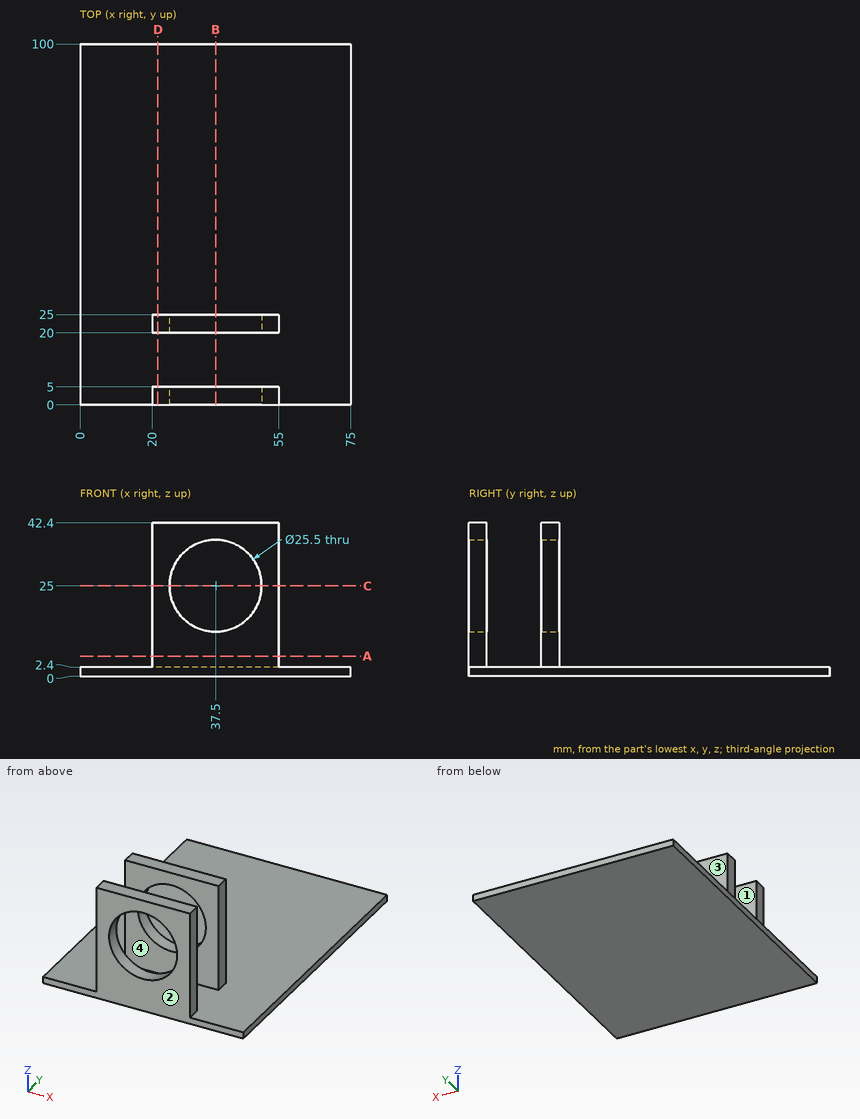
Geometry: see drawing. Coordinates: mm, zero at the bounding-box minimum. Coordinates: 2 decimals unless noted, no trailing zeros. Loops run counter-clockwise (first coordinate to the right, second up) from the corner with the lowest first, then second, coordinate; pieces in that order, holes last. Notation, with made-up numbers: (37, 33) -> (64, 33) arc R20 ccw to (64, 50) -> close; hole circle Ø8 at (-39, -18). An arc over 180 degrees is marked (long way). Use a Markdown table: item, result.
1) Contact query for flat-ended pins moving along their axis: pin 1 (5.5 mm diameter, centred on y = 2.5, z = 31, fed in from +X); pin 2 (22.5 mm diameter, centred on x = 20.5, y = 68, fed in from +Z); pin 3 (6 mm diameter, centred on x = 40, z = 18, fed in from +Y); pin 4 (4 mm diameter, centred on y = 22.5, z = 21.5, fed in from -X). Output: stop coordinate, or through.
Results found:
| item | result |
|---|---|
| pin 1 | stops at x = 55 |
| pin 2 | stops at z = 2.4 |
| pin 3 | passes through |
| pin 4 | stops at x = 20 |
2) Cut plane A-A (z = 5.5). Return the cut outline in (x, y).
Results found:
| item | result |
|---|---|
| outline | (20, 0) -> (55, 0) -> (55, 5) -> (20, 5) -> close; (20, 20) -> (55, 20) -> (55, 25) -> (20, 25) -> close |
3) Cut plane B-B (x = 37.5). Return the cut outline in (y, z), then the cut area to 3 significant figures.
Results found:
| item | result |
|---|---|
| outline | (0, 0) -> (100, 0) -> (100, 2.4) -> (25, 2.4) -> (25, 12.25) -> (20, 12.25) -> (20, 2.4) -> (5, 2.4) -> (5, 12.25) -> (0, 12.25) -> close; (0, 37.75) -> (5, 37.75) -> (5, 42.4) -> (0, 42.4) -> close; (20, 37.75) -> (25, 37.75) -> (25, 42.4) -> (20, 42.4) -> close |
| area | 385 mm2 |
4) Material intervals for line 1 along Z through (x, y) = (37, 1); line 2 along X through (y, z) = (22.8, 25); line 3 along Y through (x, z) = (24.5, 30.5), sorted ascending. Write a range as from..to.
Results found:
| item | result |
|---|---|
| line 1 | z = 0..12.26, 37.74..42.4 |
| line 2 | x = 20..24.75, 50.25..55 |
| line 3 | y = 0..5, 20..25 |
5) Cut plane D-D (x = 21.5). Return the cut outline in (y, z), then the cut area to 3 significant figures.
Results found:
| item | result |
|---|---|
| outline | (0, 0) -> (100, 0) -> (100, 2.4) -> (25, 2.4) -> (25, 42.4) -> (20, 42.4) -> (20, 2.4) -> (5, 2.4) -> (5, 42.4) -> (0, 42.4) -> close |
| area | 640 mm2 |
6) Cut plane C-C (z = 25). Return the cut outline in (x, y), then the cut area to 3 significant figures.
Results found:
| item | result |
|---|---|
| outline | (20, 0) -> (24.75, 0) -> (24.75, 5) -> (20, 5) -> close; (20, 20) -> (24.75, 20) -> (24.75, 25) -> (20, 25) -> close; (50.25, 0) -> (55, 0) -> (55, 5) -> (50.25, 5) -> close; (50.25, 20) -> (55, 20) -> (55, 25) -> (50.25, 25) -> close |
| area | 95.0 mm2 |
7) Pull-direction query (Y, two-part tool) for the marked faces 1, 2, 3 and 4; classes: released by +Y, released by -Y, zero draft, split by the parting line, or undercut.
Results found:
| item | result |
|---|---|
| face 1 | undercut |
| face 2 | released by -Y |
| face 3 | released by +Y |
| face 4 | undercut |
